from build123d import *

# Parameters (mm, degrees)
SKETCH_1_W               = 60.2
SKETCH_1_H               = 40.6
SKETCH_1_R               = 9.4
SKETCH_1_R_2             = 2.5
EXTRUDE_1_DEPTH          = 6
SKETCH_2_W               = 60.2
SKETCH_2_H               = 40.6
EXTRUDE_2_DEPTH          = 3.5
SKETCH_3_W               = 60.2
SKETCH_3_H               = 8.4
CUT_EXTRUDE_1_DEPTH      = 3.5
SKETCH_4_W               = 8.8
SKETCH_4_H               = 40.6
CUT_EXTRUDE_2_DEPTH      = 3.5
SKETCH_5_R               = 2.5
SKETCH_5_R_2             = 1.5
CUT_EXTRUDE_3_DEPTH      = 10
CUT_EXTRUDE_3_DEPTH_BACK = 10
FILLET_3_R               = 5
FILLET_8_R               = 5
FILLET_9_R               = 5
FILLET_10_R              = 5
FILLET_11_R              = 1
FILLET_12_R              = 1
FILLET_13_R              = 1
FILLET_14_R              = 1
FILLET_15_R              = 1
FILLET_16_R              = 1
FILLET_17_R              = 1
FILLET_18_R              = 1


with BuildPart() as part:
    # 草图1 → 凸台-拉伸1 (new body)
    with BuildSketch(Plane.XY):
        with Locations((19.7, -9.9)):
            Rectangle(SKETCH_1_W, SKETCH_1_H)
        Circle(SKETCH_1_R, mode=Mode.SUBTRACT)
        with Locations((19.8, 0)):
            Circle(SKETCH_1_R, mode=Mode.SUBTRACT)
        with Locations((39.6, 0)):
            Circle(SKETCH_1_R, mode=Mode.SUBTRACT)
        with Locations((0, -19.8)):
            Circle(SKETCH_1_R, mode=Mode.SUBTRACT)
        with Locations((19.8, -19.8)):
            Circle(SKETCH_1_R, mode=Mode.SUBTRACT)
        with Locations((39.6, -19.8)):
            Circle(SKETCH_1_R, mode=Mode.SUBTRACT)
        with Locations((9.9, -9.9)):
            Circle(SKETCH_1_R_2, mode=Mode.SUBTRACT)
        with Locations((29.7, -9.9)):
            Circle(SKETCH_1_R_2, mode=Mode.SUBTRACT)
    extrude(amount=EXTRUDE_1_DEPTH)

    # 草图2 → 凸台-拉伸2 (add)
    with BuildSketch(Plane.XY.offset(6)):
        with Locations((19.7, -9.9)):
            Rectangle(SKETCH_2_W, SKETCH_2_H)
    extrude(amount=EXTRUDE_2_DEPTH)

    # 草图3 → 切除-拉伸1 (cut)
    with BuildSketch(Plane.XY.offset(9.5)):
        with Locations((19.7, -0.18)):
            Rectangle(SKETCH_3_W, SKETCH_3_H)
        with Locations((19.7, -19.62)):
            Rectangle(SKETCH_3_W, SKETCH_3_H)
    extrude(amount=-CUT_EXTRUDE_1_DEPTH, mode=Mode.SUBTRACT)

    # 草图4 → 切除-拉伸2 (cut)
    with BuildSketch(Plane.XY.offset(9.5)):
        with Locations((0, -9.9)):
            Rectangle(SKETCH_4_W, SKETCH_4_H)
        with Locations((19.8, -9.9)):
            Rectangle(SKETCH_4_W, SKETCH_4_H)
        with Locations((39.6, -9.9)):
            Rectangle(SKETCH_4_W, SKETCH_4_H)
        with Locations((59.4, -9.9)):
            Rectangle(SKETCH_4_W, SKETCH_4_H)
    extrude(amount=-CUT_EXTRUDE_2_DEPTH, mode=Mode.SUBTRACT)

    # 草图5 → 切除-拉伸3 (cut, two sides)
    with BuildSketch(Plane(origin=(0, 0, 6), x_dir=(-1, 0, 0), z_dir=(0, 0, -1))) as cut_extrude_3_sk:
        with Locations((-29.7, -9.9)):
            Circle(SKETCH_5_R)
        with Locations((-9.9, -9.9)):
            Circle(SKETCH_5_R)
        with Locations((-46.944325479, -9.9)):
            Circle(SKETCH_5_R_2)
        with Locations((7.544325479, -9.9)):
            Circle(SKETCH_5_R_2)
    extrude(amount=CUT_EXTRUDE_3_DEPTH, mode=Mode.SUBTRACT)
    extrude(cut_extrude_3_sk.sketch, amount=-CUT_EXTRUDE_3_DEPTH_BACK, mode=Mode.SUBTRACT)

    # 圆角3
    fillet_3_edges = [part.edges().sort_by_distance(p)[0] for p in [
        (-10.4, -30.2, 4.75),
    ]]
    fillet(fillet_3_edges, radius=FILLET_3_R)

    # 圆角8
    fillet_8_edges = [part.edges().sort_by_distance(p)[0] for p in [
        (49.8, -30.2, 4.75),
    ]]
    fillet(fillet_8_edges, radius=FILLET_8_R)

    # 圆角9
    fillet_9_edges = [part.edges().sort_by_distance(p)[0] for p in [
        (49.8, 10.4, 4.75),
    ]]
    fillet(fillet_9_edges, radius=FILLET_9_R)

    # 圆角10
    fillet_10_edges = [part.edges().sort_by_distance(p)[0] for p in [
        (-10.4, 10.4, 4.75),
    ]]
    fillet(fillet_10_edges, radius=FILLET_10_R)

    # 圆角11
    fillet_11_edges = [part.edges().sort_by_distance(p)[0] for p in [
        (4.4, -4.38, 7.75),
    ]]
    fillet(fillet_11_edges, radius=FILLET_11_R)

    # 圆角12
    fillet_12_edges = [part.edges().sort_by_distance(p)[0] for p in [
        (4.4, -15.42, 7.75),
    ]]
    fillet(fillet_12_edges, radius=FILLET_12_R)

    # 圆角13
    fillet_13_edges = [part.edges().sort_by_distance(p)[0] for p in [
        (15.4, -15.42, 7.75),
    ]]
    fillet(fillet_13_edges, radius=FILLET_13_R)

    # 圆角14
    fillet_14_edges = [part.edges().sort_by_distance(p)[0] for p in [
        (15.4, -4.38, 7.75),
    ]]
    fillet(fillet_14_edges, radius=FILLET_14_R)

    # 圆角15
    fillet_15_edges = [part.edges().sort_by_distance(p)[0] for p in [
        (24.2, -15.42, 7.75),
    ]]
    fillet(fillet_15_edges, radius=FILLET_15_R)

    # 圆角16
    fillet_16_edges = [part.edges().sort_by_distance(p)[0] for p in [
        (35.2, -15.42, 7.75),
    ]]
    fillet(fillet_16_edges, radius=FILLET_16_R)

    # 圆角17
    fillet_17_edges = [part.edges().sort_by_distance(p)[0] for p in [
        (35.2, -4.38, 7.75),
    ]]
    fillet(fillet_17_edges, radius=FILLET_17_R)

    # 圆角18
    fillet_18_edges = [part.edges().sort_by_distance(p)[0] for p in [
        (24.2, -4.38, 7.75),
    ]]
    fillet(fillet_18_edges, radius=FILLET_18_R)


solid = part.part
Design review of the part built by this model. Coordinates are the model's own, in mm. A direction names the side the tool comes from. Give positions to 0.01 mm unless a question says otherwise; leave off trailing zeros. Loops run counter-clockwise (first coordinate to the right, second up) from the corner with the lowest first, then second, coordinate; pieces in that order, holes last. Notation, with made-up numbers: (-2.5, 8) - (32.5, 8) arc R19 ccw to (32.5, 12) - close; hole circle Ø1 at (26.5, -33). An arc over 180 degrees is marked (long way). Use CSV: the item, a comma, the result in double quotes. Start each with the question number.
1. Wall thickness on L1, parallel to X at y = 4, z = 5; L2, parallel to Y at x = 0, z = 2.95; L3, parallel to Y at x = -5, z = 7.75: over which ranges is each line inside the solid? List them lowest first.
2. Add section A-A (x = 19.8). State the section outline as (y, z) points.
3. Machinability: for faces 1 (the flat face through (-6, -14, 6)), 2 (the flat face through (44, -27, 8)), 3 (the flat face through (10, -20, 6)), which of the approach directions +Z, -Z, +X, -X, +Y, -Y give a long, thin tool a straight path to every point of the face, cutting with its end or side? Answer none if there is none.
4. Add section B-B (y = 0). State the section outline as (x, z) points, plus the area to 3 significant figures.
5. Draft analysis for pull direction X (two halves, no side actions). For faces 4 (the flat face through (24.2, -10, 8)), 5 (the cylindrical face through (48.3, -28.77, 4.82)), 6 (the flat face through (45, -6, 6)), 7 (the flat face through (47, 4.02, 8)), state which applies: released by +X, released by -X, zero draft, split by the parting line, or undercut.
6. Add section C-C (z = 1.5). Count the separate pieces of the cut face and the enclosed holes in it, plus the area to 3 significant figures.
7. Insertion check: P1, Ø5, axis at x = 37.5, y = -14.5, coming from the -Z side; P2, Ø3, axis at x = -1.5, y = -8, coming from the +Z side; P3, Ø1, axis at x = 48, z = 8, coming from the -Y side. Each pin has a flat end and moves straight along its axis. Give the tip position at first contact, or say it passes through.
Results found:
1,L1,"x = -10.4 to -8.51, 8.51 to 11.29, 28.31 to 31.09, 48.11 to 49.8"
1,L2,"y = -30.2 to -29.2, -10.4 to -9.4, 9.4 to 10.4"
1,L3,"y = -30.2 to -23.82, -15.42 to -4.38, 4.02 to 10.4"
2,outline,"(-30.2, 0) - (-29.2, 0) - (-29.2, 6) - (-30.2, 6) - close; (-10.4, 0) - (-9.4, 0) - (-9.4, 6) - (-10.4, 6) - close; (9.4, 0) - (10.4, 0) - (10.4, 6) - (9.4, 6) - close"
3,face 1,"-Z"
3,face 2,"+Z, +Y, -Y"
3,face 3,"+Z, +X, -X"
4,outline,"(-10.4, 0) - (-9.4, 0) - (-9.4, 6) - (-10.4, 6) - close; (9.4, 0) - (10.4, 0) - (10.4, 6) - (9.4, 6) - close; (29.2, 0) - (30.2, 0) - (30.2, 6) - (29.2, 6) - close; (49, 0) - (49.8, 0) - (49.8, 6) - (49, 6) - close"
4,area,"22.8 mm²"
5,face 4,"undercut"
5,face 5,"released by +X"
5,face 6,"undercut"
5,face 7,"zero draft"
6,separate pieces,"1"
6,enclosed holes,"10"
6,area,"704 mm²"
7,P1,"stops at z = 6"
7,P2,"stops at z = 6"
7,P3,"stops at y = -29.41"
